Design review of the part built by this model. Coordinates are the model's own, in mm. A direction names the side the tool comes from. Round coordinates to 2 decimals unless told otherwise and drop trailing zeros. Order: outer loops, then holes, each group sorted by start corner. A loop starts at its lowest first (then second) coordinate and runs counter-clockwise, first axis right, second up. Notation, with made-up numbers: M 15,75.5 L 45,75.5 A27 ccw 45,111.5 Z; hole C 64,-17 d9. An arc over 180 degrees is marked long. Use a Markdown table: item, result. Add a question column.
(1) For pin 1 (8 mm diameter, centred on x = 0, z = 0, fed in from -Y); pin 2 (2 mm diameter, centred on x = 56.5, y = 6.5, fed in from +Z); pin 3 (24 mm diameter, centred on x = -2, z = 2, fed in from -Y); pin 4 (1.9 mm diameter, centred on x = -8, z = 0.26, fed in from -Y), all flat-tipped, find the tip position at first contact; note any pin that passes through.
(2) Machinability: for faces 1 (the face through (12.26, 12.84, 29.6)), 2 (the face through (57.855, 2.958, -48.546)), 3 (the face through (-12.23, 12.84, 29.53)), which of the approach directions +Z, -Z, +X, -X, +Y, -Y give a long, thin tool a straight path to every point of the face, cutting with its end or side? Answer none if there is none.
(3) Take a section at B-B (x = 53.5). Write out the cut boundary in (y, z), then the cut area to 3 significant figures.
(4) Take a section at D-D (x = 76.5). Write out the cut boundary in (y, z), then the cut area to 3 significant figures.
(5) To check wall thickness, follow probe 1 along X at (y, z) = (23.8, 0); probe 2 along Z at (x, y) = (0, 1.05); probe 3 along Z at (x, y) = (0, 2.9). State the ranges of each line that lie inside material, in increasing order. Write a range as from..to.
(6) The part is to be moulded in two halves that separate along X. For faces 4 (the face through (-49.158, 2.958, 58.584)), 5 (the face through (8, 24.5, 6)), 6 (the face through (-31.768, 12.844, -4.182)), say which applies: released by +X, released by -X, zero draft, split by the parting line, or undercut.
(7) Take a section at C-C (z = 74). Write out the cut boundary in (x, y), then the cut area to 3 significant figures.
(8) Take a section at A-A (y = 15.25). Write out the cut boundary in (x, z), then the cut area to 3 significant figures.
```python
from build123d import *

# Parameters (mm, degrees)
SCHIZZO1_W                                          = 81
SCHIZZO1_H                                          = 6
ESTRUSIONE_ESTRUSIONE2_START                        = 13.5
ESTRUSIONE_ESTRUSIONE2_DEPTH                        = 13.5
ESTRUSIONE_ESTRUSIONE3_START                        = 5
SCHIZZO4_R                                          = 35
ESTRUSIONE_ESTRUSIONE3_DEPTH                        = 5
TAGLIA_RIVOLUZIONE2_DEPTH                           = 6
RIPETIZIONECIRCOLARE1_COUNT                         = 4
SCHIZZO6_R                                          = 11
TAGLIO_ESTRUSIONE2_DEPTH                            = 2
SCHIZZO7_R                                          = 1.6
TAGLIO_ESTRUSIONE3_DEPTH                            = 22
FORO_LAMATO_PER_VITE_M4_A_TESTA_SOTTILE_D           = 4.5
FORO_LAMATO_PER_VITE_M4_A_TESTA_SOTTILE_DEPTH       = 9
FORO_LAMATO_PER_VITE_M4_A_TESTA_SOTTILE_CBORE_D     = 10
FORO_LAMATO_PER_VITE_M4_A_TESTA_SOTTILE_CBORE_DEPTH = 4.5
FORO_LAMATO_PER_VITE_M4_A_TESTA_SOTTILE_TIP         = 1.351936393


# Read off the part's stored shape, not the designer's step: Taglia-Rivoluzione2
with BuildPart() as part:
    # Schizzo1 → Rivoluzione1 (revolve)
    with BuildSketch(Plane.XY):
        with Locations((-69.5, 3)):
            Rectangle(SCHIZZO1_W, SCHIZZO1_H)
    revolve(axis=Axis((0, 30.5, 0), (0, -1, 0)))

    # Schizzo3 → Estrusione-Estrusione2 (add)
    with BuildSketch(Plane(origin=(0, 6, 0), x_dir=(1, 0, 0), z_dir=(0, 1, 0)).offset(ESTRUSIONE_ESTRUSIONE2_START)):
        with BuildLine():
            Line((21.306650015, 27.76736691), (17.654081441, 23.007246868))
            ThreePointArc((17.654081441, 23.007246868), (25.11473671, 14.5), (28.75190098, 3.785259574))
            Line((28.75190098, 3.785259574), (34.700570148, 4.568416728))
            ThreePointArc((34.700570148, 4.568416728), (30.310889132, 17.5), (21.306650015, 27.76736691))
        make_face()
        with BuildLine():
            ThreePointArc((-21.306650015, 27.76736691), (-30.310889132, 17.5), (-34.700570148, 4.568416728))
            Line((-34.700570148, 4.568416728), (-28.75190098, 3.785259574))
            ThreePointArc((-28.75190098, 3.785259574), (-25.11473671, 14.5), (-17.654081441, 23.007246868))
            Line((-17.654081441, 23.007246868), (-21.306650015, 27.76736691))
        make_face()
        with BuildLine():
            ThreePointArc((-13.393920133, -32.335783638), (0, -35), (13.393920133, -32.335783638))
            Line((13.393920133, -32.335783638), (11.097819539, -26.792506443))
            ThreePointArc((11.097819539, -26.792506443), (0, -29), (-11.097819539, -26.792506443))
            Line((-11.097819539, -26.792506443), (-13.393920133, -32.335783638))
        make_face()
    extrude(amount=-ESTRUSIONE_ESTRUSIONE2_DEPTH)

    # Schizzo4 → Estrusione-Estrusione3 (add)
    with BuildSketch(Plane(origin=(0, 19.5, 0), x_dir=(1, 0, 0), z_dir=(0, 1, 0)).offset(ESTRUSIONE_ESTRUSIONE3_START)):
        with Locations(Location((0, 0, 0), (0, 0, 7.5))):
            Circle(SCHIZZO4_R)
    extrude(amount=-ESTRUSIONE_ESTRUSIONE3_DEPTH)

    # Taglia-Rivoluzione2 outline → Taglia-Rivoluzione2 (cut)
    with BuildSketch(Plane(origin=(0, 0, 0), x_dir=(1, 0, 0), z_dir=(0, 1, 0))):
        with BuildLine():
            Line((-84.264888743, 70.706637066), (-32.173866611, 26.997079607))
            ThreePointArc((-32.173866611, 26.997079607), (-29.69848481, 29.69848481), (-26.997079607, 32.173866611))
            Line((-26.997079607, 32.173866611), (-70.706637066, 84.264888743))
            ThreePointArc((-70.706637066, 84.264888743), (-77.781745931, 77.781745931), (-84.264888743, 70.706637066))
        make_face()
    taglia_rivoluzione2 = extrude(amount=TAGLIA_RIVOLUZIONE2_DEPTH, mode=Mode.SUBTRACT)

    # RipetizioneCircolare1: Taglia-Rivoluzione2 ×4 about axis
    ripetizionecircolare1_axis = Axis((0, 6, 0), (0, 1, 0))
    for i in range(1, RIPETIZIONECIRCOLARE1_COUNT):
        add(taglia_rivoluzione2.rotate(ripetizionecircolare1_axis, i * 360 / RIPETIZIONECIRCOLARE1_COUNT), mode=Mode.SUBTRACT)

    # Schizzo6 → Taglio-Estrusione2 (cut)
    with BuildSketch(Plane.XZ.offset(-19.5)):
        Circle(SCHIZZO6_R)
    extrude(amount=-TAGLIO_ESTRUSIONE2_DEPTH, mode=Mode.SUBTRACT)

    # Schizzo7 → Taglio-Estrusione3 (cut)
    with BuildSketch(Plane.XZ.offset(-21.5)):
        with Locations((-7.995791255, 0.259465219)):
            Circle(SCHIZZO7_R)
        with Locations((0.259465219, 7.995791255)):
            Circle(SCHIZZO7_R)
        with Locations((7.995791255, -0.259465219)):
            Circle(SCHIZZO7_R)
        with Locations((-0.259465219, -7.995791255)):
            Circle(SCHIZZO7_R)
        with BuildLine():
            Line((-1.5, -2), (1.5, -2))
            ThreePointArc((1.5, -2), (0, 2.5), (-1.5, -2))
        make_face()
    extrude(amount=-TAGLIO_ESTRUSIONE3_DEPTH, mode=Mode.SUBTRACT)

    # Foro lamato per Vite M4 a testa sottile cilindrica1
    with Locations(Plane(origin=(0, 6, 0), x_dir=(1, 0, 0), z_dir=(0, 1, 0))):
        with Locations((-103, 0), (103, 0), (0, 103), (0, -103)):
            CounterBoreHole(FORO_LAMATO_PER_VITE_M4_A_TESTA_SOTTILE_D / 2, FORO_LAMATO_PER_VITE_M4_A_TESTA_SOTTILE_CBORE_D / 2, FORO_LAMATO_PER_VITE_M4_A_TESTA_SOTTILE_CBORE_DEPTH, depth=FORO_LAMATO_PER_VITE_M4_A_TESTA_SOTTILE_DEPTH)
            with Locations((0, 0, -(FORO_LAMATO_PER_VITE_M4_A_TESTA_SOTTILE_DEPTH + FORO_LAMATO_PER_VITE_M4_A_TESTA_SOTTILE_TIP / 2))):  # 118° drill point
                Cone(0, FORO_LAMATO_PER_VITE_M4_A_TESTA_SOTTILE_D / 2, FORO_LAMATO_PER_VITE_M4_A_TESTA_SOTTILE_TIP, mode=Mode.SUBTRACT)


solid = part.part
```
Verdict:
| question | item | result |
|---|---|---|
| 1 | pin 1 | stops at y = 21.5 |
| 1 | pin 2 | stops at z = 94.89 |
| 1 | pin 3 | stops at y = 19.5 |
| 1 | pin 4 | passes through |
| 2 | face 1 | -Z, +X |
| 2 | face 2 | +Y, -Y |
| 2 | face 3 | -Z, -X |
| 3 | outline | M 0,-96.11 L 6,-96.11 L 6,-63.76 L 0,-63.76 Z; M 0,-44.89 L 6,-44.89 L 6,44.89 L 0,44.89 Z; M 0,63.76 L 6,63.76 L 6,96.11 L 0,96.11 Z |
| 3 | area | 927 mm^2 |
| 4 | outline | M 0,-64.19 L 6,-64.19 L 6,64.19 L 0,64.19 Z |
| 4 | area | 770 mm^2 |
| 5 | probe 1 | x = -35..-9.57, -6.42..-2.5, 2.5..6.42, 9.57..35 |
| 5 | probe 2 | z = -110..-105.25, -100.75..-29, 29..100.75, 105.25..110 |
| 5 | probe 3 | z = -110..-108, -98..-29, 29..98, 108..110 |
| 6 | face 4 | undercut |
| 6 | face 5 | zero draft |
| 6 | face 6 | released by -X |
| 7 | outline | M -62.09,0 L 62.09,0 L 62.09,6 L -62.09,6 Z |
| 7 | area | 745 mm^2 |
| 8 | outline | M -34.7,-4.57 A35 ccw -21.31,-27.77 L -17.65,-23.01 A29 cw -28.75,-3.79 Z; M -13.39,32.34 L -11.1,26.79 A29 cw 11.1,26.79 L 13.39,32.34 A35 ccw Z; M 17.65,-23.01 L 21.31,-27.77 A35 ccw 34.7,-4.57 L 28.75,-3.79 A29 cw Z |
| 8 | area | 452 mm^2 |
